from build123d import *

# Parameters (mm, degrees)
F0_R     = 38.1
F1_DEPTH = 12.7
F2_R     = 5.08


with BuildPart() as f1:
    # F0 (on Top) → F1 (new body)
    with BuildSketch(Plane.XY):
        with BuildLine():
            ThreePointArc((50.656924, -3.81), (50.764218, -1.906343), (50.8, 0))
            ThreePointArc((50.8, 0), (50.764218, 1.906343), (50.656924, 3.81))
            ThreePointArc((50.656924, 3.81), (48.456851, 15.250362), (43.708314, 25.888671))
            ThreePointArc((43.708314, 25.888671), (35.921024, 35.921024), (25.888671, 43.708314))
            ThreePointArc((25.888671, 43.708314), (14.94649, 48.551441), (3.175, 50.700684))
            ThreePointArc((3.175, 50.700684), (0, 50.8), (-3.175, 50.700684))
            ThreePointArc((-3.175, 50.700684), (-36.145183, 35.695458), (-50.73646, 2.54))
            ThreePointArc((-50.73646, 2.54), (-50.8, 0), (-50.73646, -2.54))
            ThreePointArc((-50.73646, -2.54), (-48.644054, -14.642269), (-43.708314, -25.888671))
            ThreePointArc((-43.708314, -25.888671), (-35.921024, -35.921024), (-25.888671, -43.708314))
            ThreePointArc((-25.888671, -43.708314), (-14.337666, -48.734704), (-1.905, -50.764269))
            ThreePointArc((-1.905, -50.764269), (0, -50.8), (1.905, -50.764269))
            ThreePointArc((1.905, -50.764269), (35.240102, -36.589277), (50.656924, -3.81))
        make_face()
        Circle(F0_R, mode=Mode.SUBTRACT)
        with BuildLine():
            ThreePointArc((50.656924, 3.81), (50.764218, 1.906343), (50.8, 0))
            ThreePointArc((50.8, 0), (50.764218, -1.906343), (50.656924, -3.81))
            Line((50.656924, -3.81), (55.88, -3.81))
            Line((55.88, -3.81), (55.88, 3.81))
            Line((55.88, 3.81), (50.656924, 3.81))
        make_face()
        with BuildLine():
            ThreePointArc((25.888671, 43.708314), (35.921024, 35.921024), (43.708314, 25.888671))
            ThreePointArc((43.708314, 25.888671), (47.804199, 31.439935), (48.393645, 38.31346))
            ThreePointArc((48.393645, 38.31346), (40.798679, 39.986856), (40.520196, 47.758998))
            ThreePointArc((40.520196, 47.758998), (32.532533, 48.160637), (25.888671, 43.708314))
        make_face()
        with BuildLine():
            Line((1.905, -55.88), (1.905, -50.764269))
            ThreePointArc((1.905, -50.764269), (0, -50.8), (-1.905, -50.764269))
            Line((-1.905, -50.764269), (-1.905, -55.88))
            Line((-1.905, -55.88), (1.905, -55.88))
        make_face()
        with BuildLine():
            ThreePointArc((-3.175, 50.700684), (0, 50.8), (3.175, 50.700684))
            Line((3.175, 50.700684), (3.175, 55.88))
            Line((3.175, 55.88), (-3.175, 55.88))
            Line((-3.175, 55.88), (-3.175, 50.700684))
        make_face()
        with BuildLine():
            ThreePointArc((-40.520196, -47.758998), (-32.532533, -48.160637), (-25.888671, -43.708314))
            ThreePointArc((-25.888671, -43.708314), (-35.921024, -35.921024), (-43.708314, -25.888671))
            ThreePointArc((-43.708314, -25.888671), (-47.804199, -31.439935), (-48.393645, -38.31346))
            ThreePointArc((-48.393645, -38.31346), (-40.798679, -39.986856), (-40.520196, -47.758998))
        make_face()
        with BuildLine():
            ThreePointArc((-50.73646, -2.54), (-50.8, 0), (-50.73646, 2.54))
            Line((-50.73646, 2.54), (-55.88, 2.54))
            Line((-55.88, 2.54), (-55.88, -2.54))
            Line((-55.88, -2.54), (-50.73646, -2.54))
        make_face()
    extrude(amount=F1_DEPTH)

    # F2
    f2_edges = [f1.edges().sort_by_distance(p)[0] for p in [
        (-48.393645, -38.31346, 6.35),
        (-40.520196, -47.758998, 6.35),
        (40.520196, 47.758998, 6.35),
        (48.393645, 38.31346, 6.35),
    ]]
    fillet(f2_edges, radius=F2_R)


solid = f1.part
Geometry: final body of the model. Coordinates: model frame, mm. A direction names the side the tool comes from. Give positions to 0.01 mm unless a question says otherwise; leave off trailing zeros. Write each loop counter-clockwise with the first axis right and the second up, starting at its lowest first coordinate (ties: lowest second). Pieces come first, ordered by that corner, then holes.
(1) Mould query, pull axis Y, two halves, no side actions, for faces 1 (the cylindrical face through (-35.78, 36.06, 6.26)), 2 (the cylindrical face through (-48.693, -14.477, 6.261)), 3 (the flat face through (0, -55.88, 6)), 4 (the flat face through (-1.905, -53, 6)). Classes: released by +Y, released by -Y, zero draft, split by the parting line, or undercut.
(2) Access query for faces 5 (the flat face through (-53, -2.54, 6)), 6 (the flat face through (-3.175, 53, 6)), 7 (the cylindrical face through (-14.507, -48.685, 6.261)), 8 (the cylindrical face through (45.963, 28.146, 6.261)), 9 (the cylindrical face through (-45.963, -28.146, 6.261)). Directions: +Z, -Z, +X, -X, +Y, -Y. A direction counts if a zero-diameter tool reaches every point of the face in a straight line with its end or side. Return the directions, or none.
(3) Cut plane A-A, the plane x = 0. Return loops of the section in (y, z).
(4) First-contact query: P1, Ø1.6, axis at x = 54.5, z = 4.5, coming from the -Y side; P2, Ø5, axis at x = 44.5, z = 6, coming from the -Y side; P3, Ø4, axis at y = 53.5, z = 9.5, coming from the -X side (3 decimals). Flat tips, straight axial feed; report the tip coordinate or a pass-through.
(5) Ray query, line 1 (Y direction, x = 0, z = 2.5); line 2 (X direction, y = 9.5, z = 8.75); line 3 (Y direction, x = 16.5, z = 7.5). Return the intervals inside material, ascending.
Values follow:
1. face 1: released by +Y
1. face 2: undercut
1. face 3: released by -Y
1. face 4: zero draft
2. face 5: +Z, -Z, -X, -Y
2. face 6: +Z, -Z, -X, +Y
2. face 7: +Z, -Z, -Y
2. face 8: +Z, -Z, +X
2. face 9: +Z, -Z, -X
3. outline: (-55.88, 0) - (-38.1, 0) - (-38.1, 12.7) - (-55.88, 12.7) - close; (38.1, 0) - (55.88, 0) - (55.88, 12.7) - (38.1, 12.7) - close
4. P1: stops at y = -3.81
4. P2: stops at y = -28.58
4. P3: stops at x = -3.175
5. line 1: y = -55.88 to -38.1, 38.1 to 55.88
5. line 2: x = -49.9 to -36.9, 36.9 to 49.9
5. line 3: y = -48.05 to -34.34, 34.34 to 48.05
